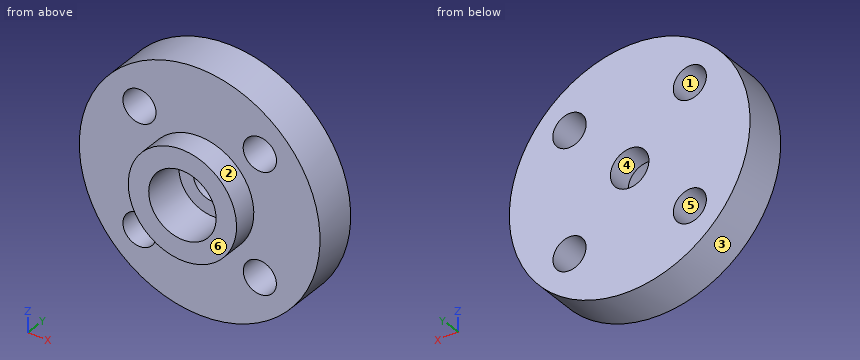
from build123d import *

# Parameters (mm, degrees)
SKETCH1_R           = 10
SKETCH1_R_2         = 1.6
SKETCH1_R_3         = 1.375
SKETCH1_R_4         = 1.386376747
BOSS_EXTRUDE1_DEPTH = 3.55
SKETCH2_W           = 1.7
SKETCH2_H           = 3.5
CUT_EXTRUDE1_START  = -1.5
SKETCH3_R           = 2.8
CUT_EXTRUDE1_DEPTH  = 1.5


with BuildPart() as part:
    # Sketch1 → Boss-Extrude1 (new body)
    with BuildSketch(Plane(origin=(0, 0, 0), x_dir=(1, 0, 0), z_dir=(0, 1, 0))):
        with Locations(Location((0, 0, 0), (0, 0, 270))):
            Circle(SKETCH1_R)
        with Locations(Location((0, 0, 0), (0, 0, 270))):
            Circle(SKETCH1_R_2, mode=Mode.SUBTRACT)
        with Locations(Location((-5, -5, 0), (0, 0, 270))):
            Circle(SKETCH1_R_3, mode=Mode.SUBTRACT)
        with Locations(Location((5, -5, 0), (0, 0, 270))):
            Circle(SKETCH1_R_4, mode=Mode.SUBTRACT)
        with Locations(Location((5, 5, 0), (0, 0, 270))):
            Circle(SKETCH1_R_3, mode=Mode.SUBTRACT)
        with Locations(Location((-5, 5, 0), (0, 0, 270))):
            Circle(SKETCH1_R_3, mode=Mode.SUBTRACT)
    extrude(amount=BOSS_EXTRUDE1_DEPTH)

    # Sketch2 → Revolve1 (revolve)
    with BuildSketch(Plane.XY, mode=Mode.PRIVATE) as revolve1_sk:
        with Locations((-3.65, -0.25)):
            Rectangle(SKETCH2_W, SKETCH2_H)
    revolve(revolve1_sk.sketch.rotate(Axis((0, 0, 0), (0, -1, 0)), 270), axis=Axis((0, 0, 0), (0, -1, 0)))

    # Sketch3 → Cut-Extrude1 (cut)
    with BuildSketch(Plane.XZ.offset(CUT_EXTRUDE1_START)):
        with Locations(Location((0, 0, 0), (0, 0, 90))):
            Circle(SKETCH3_R)
    extrude(amount=CUT_EXTRUDE1_DEPTH, mode=Mode.SUBTRACT)


solid = part.part
Read the model definition and answer for the solid it produces. Units are mm, in the model's axes. Face numbers are marked on the shaded views. A direction names the side the tool comes from. Coordinates: 2 decimals unless noted, no trailing zeros. Order: outer loops, then holes, each group sorted by start corner. A loop starts at its lowest first (then second) coordinate and runs counter-clockwise, first axis right, second up. Notation, with made-up numbers: M -13.75,-3.75 L 26.25,-3.75 A20 cw 26.25,19.25 Z; hole C 80,-14 d9. An arc over 180 degrees is marked long. Put each result on its own line as item: value. Start each with the question number.
Item 1: Consider probe 1 along X at (y, z) = (-1.1, 0); probe 2 along X at (y, z) = (2, 0); probe 3 along X at (y, z) = (1.9, -4.25). Determine where each line is inside the solid, lowest interval first. Write a range as [from, to].
Item 2: Section C-C, the plane x = -5 is taken. Determine the outline of the cut face in (y, z) (3 decimals).
Item 3: Section D-D, the plane z = 5 is taken. Determine the outline of the cut face in (x, y) (3 decimals), plus the area to 3 significant figures.
Item 4: Given pin 1 Ø1 at (x, z) = (3, 7) entering from -Y; pin 2 Ø3 at (x, z) = (0.5, 0) entering from -Y; pin 3 Ø1.5 at (y, z) = (0, -1) entering from +X, each flat-ended and moving along its own axis, determine where each tip first touches the part or whether it passes through.
Item 5: For the marked faces 1 and 2, determine the directions among +Z, -Z, +X, -X, +Y, -Y from which every point of the face is accessible in a straight line to the end or side of a thin tool.
Item 6: The mould has two halves that part along Z. Classify the marked faces 3, 4, 5 and 6: +Z half, -Z half, draft (parallel to the pull), parting line (faces both ways), or undercut.
Item 7: Section B-B, the plane y = 2.6 is taken. Determine the outline of the cut face in (x, z) (3 decimals).
Item 8: Section A-A, the plane x = 0 is taken. Determine the outline of the cut face in (y, z).
Computed:
1. probe 1: x = [-4.5, -2.8], [2.8, 4.5]
1. probe 2: x = [-10, -1.6], [1.6, 10]
1. probe 3: x = [-9.05, -6.15], [-3.85, 3.85], [6.15, 9.05]
2. outline: M 0,-8.66 L 3.55,-8.66 L 3.55,-6.375 L 0,-6.375 Z; M 0,-3.625 L 3.55,-3.625 L 3.55,3.625 L 0,3.625 Z; M 0,6.375 L 3.55,6.375 L 3.55,8.66 L 0,8.66 Z
3. outline: M -8.66,0 L -6.375,0 L -6.375,3.55 L -8.66,3.55 Z; M -3.625,0 L 3.614,0 L 3.614,3.55 L -3.625,3.55 Z; M 6.386,0 L 8.66,0 L 8.66,3.55 L 6.386,3.55 Z
3. area: 41.9 mm2
4. pin 1: stops at y = 0
4. pin 2: stops at y = 1.5
4. pin 3: stops at x = 10
5. face 1: +Y, -Y
5. face 2: -Y
6. face 3: parting line
6. face 4: undercut
6. face 5: undercut
6. face 6: draft
7. outline: C 0,0 d20; hole C -5,-5 d2.75; hole C -5,5 d2.75; hole C 0,0 d3.2; hole C 5,5 d2.773; hole C 5,-5 d2.75
8. outline: M -2,-4.5 L 0,-4.5 L 0,-10 L 3.55,-10 L 3.55,-1.6 L 1.5,-1.6 L 1.5,-2.8 L -2,-2.8 Z; M -2,2.8 L 1.5,2.8 L 1.5,1.6 L 3.55,1.6 L 3.55,10 L 0,10 L 0,4.5 L -2,4.5 Z
